Here's how the part is built. I have some questions about the finished solid (model axes, mm). Round coordinates to 2 decimals unless told otherwise and drop trailing zeros. Loops run counter-clockwise (first coordinate to the right, second up) from the corner with the lowest first, then second, coordinate; pieces in that order, holes last. Notation, with made-up numbers: M 83,50 L 123,50 A33 ccw 123,78 Z; hole C -19.75,-21.5 d10. An arc over 180 degrees is marked long. Use a Markdown table: item, result.
Autodesk Inventor part; units mm, degrees
ref_plane "YZ Plane" through (0, 0, 0) normal (1, 0, 0) x (0, 1, 0)
ref_plane "XZ Plane" through (0, 0, 0) normal (0, 1, 0) x (-1, 0, 0)
ref_plane "XY Plane" through (0, 0, 0) normal (0, 0, 1) x (1, 0, 0)
sketch "スケッチ1" plane through (0, 0, 0) normal (0, 0, 1) x (1, 0, 0)
  circle A0 centre (0, 0) radius 10.5
  circle A1 centre (0, 0) radius 5.05
  circle A2 centre (0, 8.5) radius 1.35
  circle A3 centre (-6.0104, 6.0104) radius 1.04
  line L0 (0, 8.5) -> (0, 0) construction
  line L1 (0, 0) -> (-6.0104, 6.0104) construction
  circle A4 centre (0, 0) radius 8.5 construction
  circle A5 centre (-8.5, 0) radius 1.35
  circle A6 centre (-6.0104, -6.0104) radius 1.04
  circle A7 centre (0, -8.5) radius 1.35
  circle A8 centre (6.0104, -6.0104) radius 1.04
  circle A9 centre (8.5, 0) radius 1.35
  circle A10 centre (6.0104, 6.0104) radius 1.04
  dimension "d0" = 21
  dimension "d1" = 10.1
  dimension "d2" = 2.7
  dimension "d3" = 45
  dimension "d4" = 2.08
  dimension "d5" = 17
  dimension "d8" = 360
extrude "押し出し1" add sketch "スケッチ1" along normal blind 4 contours A0 | A3 | A6 | A8 | A10
sketch "スケッチ2" plane through (0, 0, 4) normal (0, 0, 1) x (1, 0, 0)
  circle A0 centre (0, 0) radius 5.05
  circle A1 centre (0, 0) radius 10.5
  circle A2 centre (0, 0) radius 5.5
  dimension "d12" = 11
extrude "押し出し2" add sketch "スケッチ2" along normal blind 1 contours A2
sketch "スケッチ4" plane through (0, 0, 4) normal (0, 0, 1) x (1, 0, 0)
  circle A0 centre (0, 0) radius 5.5
  circle A1 centre (-8.5, 0) radius 1.35
  circle A2 centre (0, 8.5) radius 1.35
  circle A3 centre (0, 0) radius 10.5
  line L0 (0, 8.5) -> (0, 0) construction
  line L1 (0, 0) -> (-8.5, 0) construction
  line L2 (0, 0) -> (-7.4246, 7.4246) construction
  circle A4 centre (0, 0) radius 10.5 construction
  line L3 (-12.2474, 2.5) -> (-6, 2.5)
  line L4 (-2.5, 6) -> (-2.5, 12.2474)
  arc A5 (-2.5, 12.2474) -> (-12.2474, 2.5) centre (0, 0) ccw
  arc A6 (-2.5, 6) -> (-6, 2.5) centre (0, 0) ccw
  circle A7 centre (0, 0) radius 5.5
  line L5 (-2.5, -12.2474) -> (-2.5, -6)
  line L6 (-6, -2.5) -> (-12.2474, -2.5)
  arc A8 (-12.2474, -2.5) -> (-2.5, -12.2474) centre (0, 0) ccw
  arc A9 (-6, -2.5) -> (-2.5, -6) centre (0, 0) ccw
  line L7 (12.2474, -2.5) -> (6, -2.5)
  line L8 (2.5, -6) -> (2.5, -12.2474)
  arc A10 (2.5, -12.2474) -> (12.2474, -2.5) centre (0, 0) ccw
  arc A11 (2.5, -6) -> (6, -2.5) centre (0, 0) ccw
  line L9 (2.5, 12.2474) -> (2.5, 6)
  line L10 (6, 2.5) -> (12.2474, 2.5)
  arc A12 (12.2474, 2.5) -> (2.5, 12.2474) centre (0, 0) ccw
  arc A13 (6, 2.5) -> (2.5, 6) centre (0, 0) ccw
  dimension "d24" = 45
  dimension "d25" = 2.5
  dimension "d26" = 2.5
  dimension "d27" = 2
  dimension "d30" = 360
  dimension "d35" = 1
extrude "押し出し4" cut sketch "スケッチ4" against normal blind 10 contours L10 A13 L9 A3 | A3 L9 A12 L10 | L7 A10 L8 A3 | A3 L8 A11 L7 | L4 A6 L3 A3 | A3 L3 A5 L4 | L5 A8 L6 A3 | A3 L6 A9 L5
fillet "フィレット2" radius 2.5 15 edges at (2.5, -6, 2) (2.5, -10.198, 2) (-2.5, -10.198, 2) (-2.5, -6, 2) (6, -2.5, 2) (6, 2.5, 2) (10.198, -2.5, 2) (10.198, 2.5, 2) (2.5, 10.198, 2) (-2.5, 10.198, 2) (-2.5, 6, 2) (-6, 2.5, 2) (-10.198, -2.5, 2) (-10.198, 2.5, 2) (-6, -2.5, 2)
equation "\"d26\" = d25"
properties part number "リンク_ふくらはぎ_サブフレーム_1_4" material "アルミニウム 2014-T4"
1. Imagine slicing it at B-B, the plane x = -8.25. Write out the boundary of the cut face in (y, z).
Answer sheet:
| item | result |
|---|---|
| outline | M -2.49,0 L -1.33,0 L -1.33,4 L -2.49,4 Z; M 1.33,0 L 2.49,0 L 2.49,4 L 1.33,4 Z |
2. Imagine slicing it at D-D, the plane z = 2. State how many separate pieces and enclosed holes the cut face has, then the cut area to 3 significant figures.
Answer sheet:
| item | result |
|---|---|
| separate pieces | 1 |
| enclosed holes | 5 |
| area | 105 mm2 |
3. For pin 1 Ø2 at (x, y) = (8.5, 0) entering from -Z; pin 2 Ø0.6 at (y, z) = (7.5, 3) entering from -X; pin 3 Ø1 at (y, z) = (7, 3) entering from +X; pin 4 Ø2 at (y, z) = (7.5, 2.5) entering from -X, each with a flat end and sliding along its axis, tell me the tip position at first contact or that it passes through.
Answer sheet:
| item | result |
|---|---|
| pin 1 | through |
| pin 2 | x = -2.52 |
| pin 3 | x = 2.5 |
| pin 4 | x = -2.7 |
4. I need wall thicknesses on probe 1 along Y at (x, z) = (0, 1.95); probe 2 along X at (y, z) = (-0.5, 1.85); probe 3 along X at (y, z) = (-3.75, 2.25). Which ranges of each line are inside material? Lowest first, please. Write a range as from..to.
Answer sheet:
| item | result |
|---|---|
| probe 1 | -10.5..-9.85, -7.15..-5.05, 5.05..7.15, 9.85..10.5 |
| probe 2 | -10.45..-9.75, -7.25..-5.03, 5.03..7.25, 9.75..10.45 |
| probe 3 | -5.31..-3.38, 3.38..5.31 |
5. Imagine slicing it at C-C, the plane y = -0.5. Write out the boundary of the cut face in (x, z), then the cut area to 3 significant figures.
Answer sheet:
| item | result |
|---|---|
| outline | M -10.45,0 L -9.75,0 L -9.75,4 L -10.45,4 Z; M -7.25,0 L -5.03,0 L -5.03,5 L -5.48,5 L -5.48,4 L -7.25,4 Z; M 5.03,0 L 7.25,0 L 7.25,4 L 5.48,4 L 5.48,5 L 5.03,5 Z; M 9.75,0 L 10.45,0 L 10.45,4 L 9.75,4 Z |
| area | 24.2 mm2 |
6. Imagine slicing it at A-A, the plane y = -8.5. Write out the boundary of the cut face in (x, z), then the cut area to 3 significant figures.
Answer sheet:
| item | result |
|---|---|
| outline | M -2.45,0 L -1.35,0 L -1.35,4 L -2.45,4 Z; M 1.35,0 L 2.45,0 L 2.45,4 L 1.35,4 Z |
| area | 8.80 mm2 |
7. We'd pull the mould along X, two halves only. Please class faces 1 (the face through (-9.748, -1.787, 1.972)), 2 (the face through (2.5, 7, 2)), 3 (the face through (-7.212, -0.406, 1.972)): +X half, -X half, draft (parallel to the pull), parting line (faces both ways), or undercut.
Answer sheet:
| item | result |
|---|---|
| face 1 | -X half |
| face 2 | +X half |
| face 3 | undercut |
